Source: CAD feature listing. Evaluate the final solid. Frame: model axes, mm. Face numbers are marked on the shaded views. A direction names the side the tool comes from. Round coordinates to 2 decimals unless told otherwise and drop trailing zeros. Loops run counter-clockwise (first coordinate to the right, second up) from the corner with the lowest first, then second, coordinate; pieces in that order, holes last. Notation, with made-up numbers: (-9.5, -22.75) -> (14.5, -22.75) arc R32 cw to (14.5, 7.25) -> close; hole circle Ø8 at (23.5, -15.5). An arc over 180 degrees is marked (long way). Put each result on its own line as item: value. Start each with the question number.
1. Cut plane B-B (z = 12). State how many separate pieces and enclosed holes the cut face has, then the cut area to 3 significant figures.
2. Contact query for flat-ended pins moving along their axis: pin 1 (3 mm diameter, centred on x = -3, y = -11.5, fed in from +Z); pin 2 (1.3 mm diameter, centred on x = 8, y = -14, fed in from +Z); pin 3 (1.3 mm diameter, centred on x = 7.5, z = 11, fed in from -Y); pin 4 (5 mm diameter, centred on y = -3, z = 11, fed in from -X). Output: stop coordinate, or through.
3. Cut plane A-A (x = -5.5). Return the cut outline in (y, z), then the cut area to 3 significant figures.
4. Set-up query: the marked faces 1, 2, 3 and 4. Return all of +Z, -Z, +X, -X, +Y, -Y with unobstructed straight access to the full face (end or side cutting, diameter ignored); none if empty.
5. Cut plane C-C (x = 2). Return the cut outline in (y, z), then the cut area to 3 significant figures.
6. Material intervals for L1, parallel to Y at x = -12.5, z = 9; L2, parallel to Z at x = 22.5, y = -22; L3, parallel to Y at x = 6, z = 12.5, sorted ascending.
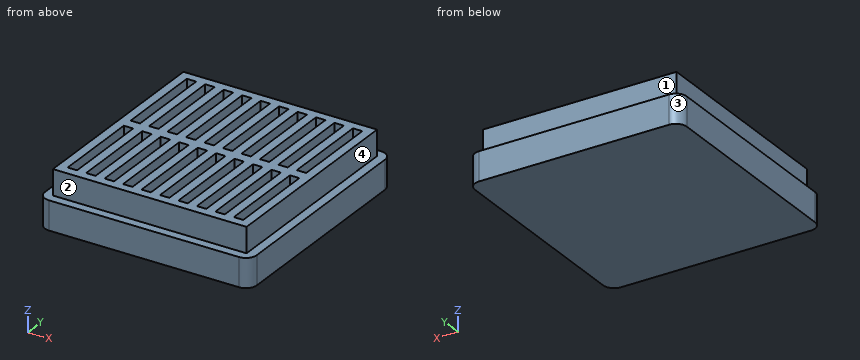
```python
from build123d import *

# Parameters (mm, degrees)
SKETCH_1_W            = 58.5
SKETCH_1_H            = 62
EXTRUDE_1_DEPTH       = 15
SKETCH_2_W            = 58.5
SKETCH_2_H            = 62
SKETCH_2_W_2          = 53.5
SKETCH_2_H_2          = 57
CUT_EXTRUDE_1_DEPTH   = 7
SKETCH_3_W            = 2.6
SKETCH_3_H            = 24.5
CUT_EXTRUDE_1_2_DEPTH = 12
FILLET_1_R            = 3


with BuildPart() as part:
    # Эскиз1 → Бобышка-Вытянуть1 (new body)
    with BuildSketch(Plane.XY):
        Rectangle(SKETCH_1_W, SKETCH_1_H)
    extrude(amount=EXTRUDE_1_DEPTH)

    # Эскиз2 → Cut-Extrude 1 (cut)
    with BuildSketch(Plane.XY.offset(15)):
        Rectangle(SKETCH_2_W, SKETCH_2_H)
        Rectangle(SKETCH_2_W_2, SKETCH_2_H_2, mode=Mode.SUBTRACT)
    extrude(amount=-CUT_EXTRUDE_1_DEPTH, mode=Mode.SUBTRACT)

    # Эскиз3 → Cut-Extrude 1 2 (cut)
    with BuildSketch(Plane.XY.offset(15)):
        with Locations((2.55, 13.75)):
            Rectangle(SKETCH_3_W, SKETCH_3_H)
        with Locations((-2.55, 13.75)):
            Rectangle(SKETCH_3_W, SKETCH_3_H)
        with Locations((7.65, 13.75)):
            Rectangle(SKETCH_3_W, SKETCH_3_H)
        with Locations((12.75, 13.75)):
            Rectangle(SKETCH_3_W, SKETCH_3_H)
        with Locations((17.85, 13.75)):
            Rectangle(SKETCH_3_W, SKETCH_3_H)
        with Locations((22.95, 13.75)):
            Rectangle(SKETCH_3_W, SKETCH_3_H)
        with Locations((-7.65, 13.75)):
            Rectangle(SKETCH_3_W, SKETCH_3_H)
        with Locations((-12.75, 13.75)):
            Rectangle(SKETCH_3_W, SKETCH_3_H)
        with Locations((-17.85, 13.75)):
            Rectangle(SKETCH_3_W, SKETCH_3_H)
        with Locations((-22.95, 13.75)):
            Rectangle(SKETCH_3_W, SKETCH_3_H)
        with Locations((22.95, -13.75)):
            Rectangle(SKETCH_3_W, SKETCH_3_H)
        with Locations((17.85, -13.75)):
            Rectangle(SKETCH_3_W, SKETCH_3_H)
        with Locations((12.75, -13.75)):
            Rectangle(SKETCH_3_W, SKETCH_3_H)
        with Locations((7.65, -13.75)):
            Rectangle(SKETCH_3_W, SKETCH_3_H)
        with Locations((2.55, -13.75)):
            Rectangle(SKETCH_3_W, SKETCH_3_H)
        with Locations((-2.55, -13.75)):
            Rectangle(SKETCH_3_W, SKETCH_3_H)
        with Locations((-7.65, -13.75)):
            Rectangle(SKETCH_3_W, SKETCH_3_H)
        with Locations((-12.75, -13.75)):
            Rectangle(SKETCH_3_W, SKETCH_3_H)
        with Locations((-17.85, -13.75)):
            Rectangle(SKETCH_3_W, SKETCH_3_H)
        with Locations((-22.95, -13.75)):
            Rectangle(SKETCH_3_W, SKETCH_3_H)
    extrude(amount=-CUT_EXTRUDE_1_2_DEPTH, mode=Mode.SUBTRACT)

    # Скругление1
    fillet_1_edges = [part.edges().sort_by_distance(p)[0] for p in [
        (29.25, -31, 4),
        (-29.25, -31, 4),
        (-29.25, 31, 4),
        (29.25, 31, 4),
    ]]
    fillet(fillet_1_edges, radius=FILLET_1_R)


solid = part.part
```
Solution:
1. separate pieces: 1
1. enclosed holes: 20
1. area: 1,780 mm^2
2. pin 1: stops at z = 15
2. pin 2: stops at z = 3
2. pin 3: stops at y = -28.5
2. pin 4: stops at x = -26.75
3. outline: (-31, 0) -> (31, 0) -> (31, 8) -> (28.5, 8) -> (28.5, 15) -> (-28.5, 15) -> (-28.5, 8) -> (-31, 8) -> close
3. area: 895 mm^2
4. face 1: +Z, +X, -X, +Y
4. face 2: +Z, +X, -X, -Y
4. face 3: +Z, -Z, -X, +Y
4. face 4: +Z, +X, +Y, -Y
5. outline: (-31, 0) -> (31, 0) -> (31, 8) -> (28.5, 8) -> (28.5, 15) -> (26, 15) -> (26, 3) -> (1.5, 3) -> (1.5, 15) -> (-1.5, 15) -> (-1.5, 3) -> (-26, 3) -> (-26, 15) -> (-28.5, 15) -> (-28.5, 8) -> (-31, 8) -> close
5. area: 307 mm^2
6. L1: y = -28.5 to -26, -1.5 to 1.5, 26 to 28.5
6. L2: z = 0 to 3
6. L3: y = -28.5 to 28.5
